Input: dimensioned drawing with shaded views. Units: mm. Origin: part minimum x, y, z. A direction names the side the tool comes from. Round coordinates to 2 decimals unless told otherwise and drop trailing zeros. Loops run counter-clockwise (first coordinate to the right, second up) from the corner with the lowest first, then second, coordinate; pieces in that order, holes last. Notation, with made-up numbers: M -8,-6.75 L 45,-6.75 A16 ccw 45,8.25 Z; hole C 62.5,57.5 d8. An arc over 180 degrees is marked long. Write each question's results on one line, items separated by ' | '. Start each with the question number.
1. Section D-D on z = 2.25. Output: boundary loops of the cut face in (x, y).
2. Ray query, line 1 (Y direction, x = 5, z = 25.7); line 2 (Z direction, x = 40, y = 34); line 3 (X direction, y = 13.5, z = 10.25). Return the intervals inside material, ascending.
3. Section C-C on y = 17.5. Output: boundary loops of the cut face in (x, z).
4. Set-up query: the marked faces 1, 2 and 3. Return all of +Z, -Z, +X, -X, +Y, -Y with unobstructed straight access to the full face (end or side cutting, diameter ignored); none if empty.
5. Contact query for flat-ended pins moving along their axis: pin 1 Ø3.5 at (x, y) = (5, 55.59) entering from -Z; pin 2 Ø3 at (y, z) = (15.5, 10) entering from +X. Output: stop coordinate, or through.
6. Section B-B on z = 14.39. Output: boundary loops of the cut face in (x, y).
7. Section A-A on x = 5. Output: boundary loops of the cut face in (y, z).
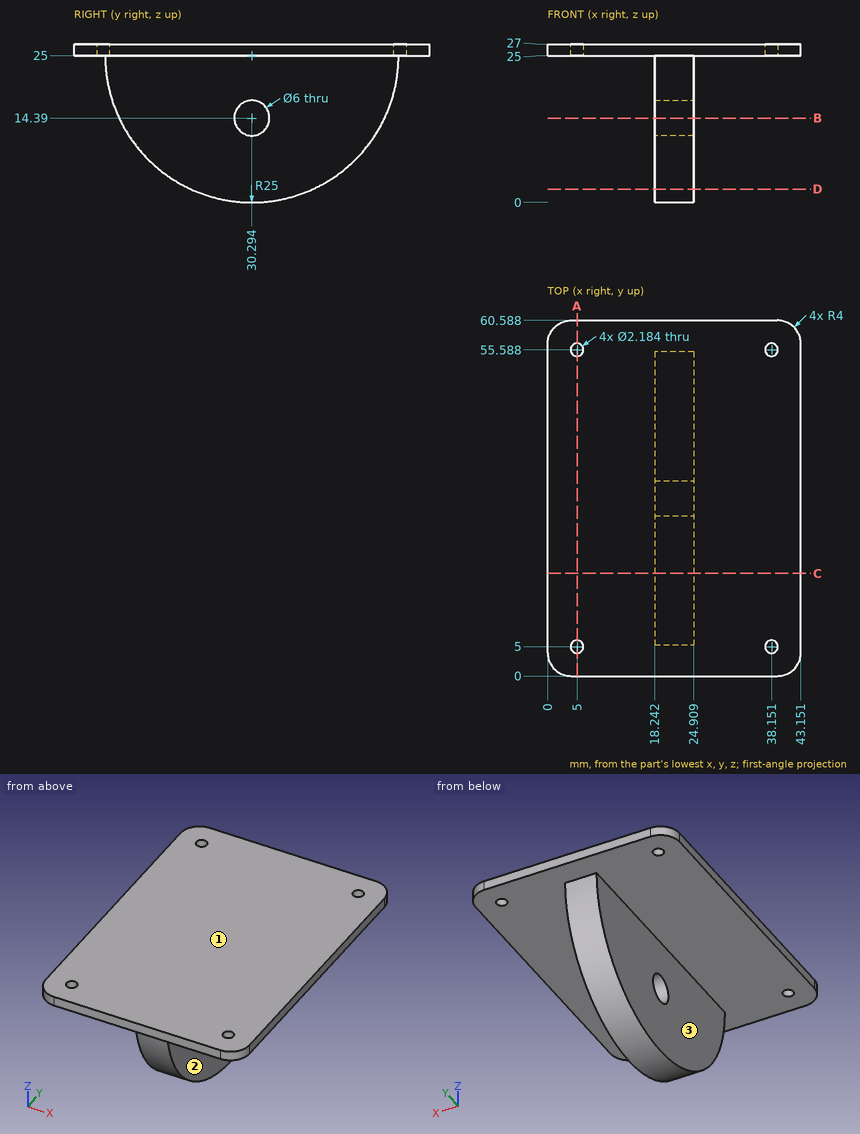
Taken from the geometry:
1) outline: M 18.24,19.93 L 24.91,19.93 L 24.91,40.66 L 18.24,40.66 Z
2) line 1: 0 to 3.91, 6.09 to 54.5, 56.68 to 60.59 | line 2: 25 to 27 | line 3: 18.24 to 24.91
3) outline: M 0,25 L 18.24,25 L 18.24,3.52 L 24.91,3.52 L 24.91,25 L 43.15,25 L 43.15,27 L 0,27 Z
4) face 1: +Z, +X, -X, +Y, -Y | face 2: -Z, +X, +Y, -Y | face 3: -Z, -X, +Y, -Y
5) pin 1: z = 25 | pin 2: x = 24.91
6) outline: M 18.24,7.66 L 24.91,7.66 L 24.91,27.29 L 18.24,27.29 Z; M 18.24,33.29 L 24.91,33.29 L 24.91,52.93 L 18.24,52.93 Z
7) outline: M 0,25 L 3.91,25 L 3.91,27 L 0,27 Z; M 6.09,25 L 54.5,25 L 54.5,27 L 6.09,27 Z; M 56.68,25 L 60.59,25 L 60.59,27 L 56.68,27 Z
